Can you work these out from the model? Positions are in its coordinate system, mm. Face numbers are marked on the shaded views. A direction names the side the tool comes from. Give positions to 0.01 mm unless a question says otherwise; leave off trailing zeros. Write each loop counter-clockwise with the first axis right and the second up, starting at its lowest first coordinate (ties: lowest second). Pieces come first, ordered by that corner, then holes.
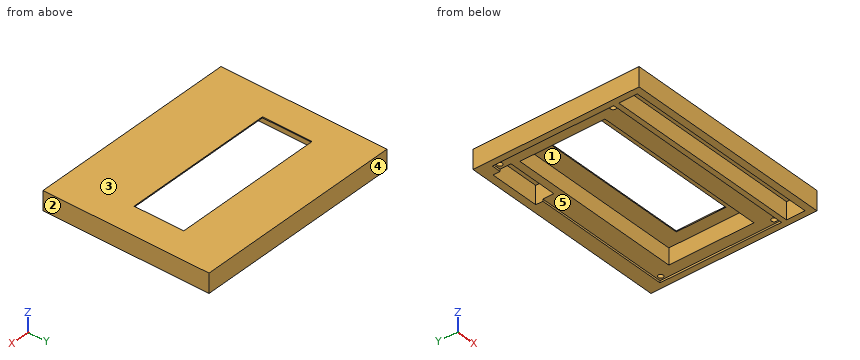
```python
from build123d import *

# Parameters (mm, degrees)
F1_W     = 104
F1_H     = 82
F1_W_2   = 87
F1_H_2   = 42
F1_W_3   = 75
F1_H_3   = 24.5
F1_W_4   = 25
F1_H_4   = 5.41
F1_H_5   = 3.5
F2_DEPTH = 9.5
F3_DEPTH = 9
F4_DEPTH = 1
F0_R     = 1.25
F5_DEPTH = 4
F6_W     = 98
F6_H     = 9.1468319297
F7_DEPTH = 8.5


with BuildPart() as f2:
    # F1 (on Top) → F2 (new body)
    with BuildSketch(Plane.XY):
        with Locations((0, -4)):
            Rectangle(F1_W, F1_H)
        Polygon((-44.4778376818, 30), (-44.4778376818, 33.5), (-19.4778376818, 33.5), (-19.4778376818, 30), (49, 30), (49, -30), (-49, -30), (-49, 30), align=None, mode=Mode.SUBTRACT)
        Polygon((-44.4778376818, 24.59), (-44.4778376818, 30), (-49, 30), (-49, -30), (49, -30), (49, 30), (-19.4778376818, 30), (-19.4778376818, 24.59), align=None)
        Rectangle(F1_W_2, F1_H_2, mode=Mode.SUBTRACT)
        Rectangle(F1_W_2, F1_H_2)
        Rectangle(F1_W_3, F1_H_3, mode=Mode.SUBTRACT)
        with Locations((-31.9778376818, 27.295)):
            Rectangle(F1_W_4, F1_H_4)
        with Locations((-31.9778376818, 31.75)):
            Rectangle(F1_W_4, F1_H_5)
    extrude(amount=F2_DEPTH)

    # F1 (on Top) → F3 (cut)
    with BuildSketch(Plane.XY):
        Rectangle(F1_W_2, F1_H_2)
        Rectangle(F1_W_3, F1_H_3, mode=Mode.SUBTRACT)
        with Locations((-31.9778376818, 27.295)):
            Rectangle(F1_W_4, F1_H_4)
        with Locations((-31.9778376818, 31.75)):
            Rectangle(F1_W_4, F1_H_5)
    extrude(amount=F3_DEPTH, mode=Mode.SUBTRACT)

    # F1 (on Top) → F4 (cut)
    with BuildSketch(Plane.XY):
        Polygon((-44.4778376818, 24.59), (-44.4778376818, 30), (-49, 30), (-49, -30), (49, -30), (49, 30), (-19.4778376818, 30), (-19.4778376818, 24.59), align=None)
        Rectangle(F1_W_2, F1_H_2, mode=Mode.SUBTRACT)
        Rectangle(F1_W_2, F1_H_2)
        Rectangle(F1_W_3, F1_H_3, mode=Mode.SUBTRACT)
        with Locations((-31.9778376818, 27.295)):
            Rectangle(F1_W_4, F1_H_4)
    extrude(amount=F4_DEPTH, mode=Mode.SUBTRACT)

    # F0 (on Top) → F5 (cut)
    with BuildSketch(Plane.XY):
        with Locations((-47, 28)):
            Circle(F0_R)
        with Locations((47, 28)):
            Circle(F0_R)
        with Locations((47, -28)):
            Circle(F0_R)
        with Locations((-47, -28)):
            Circle(F0_R)
    extrude(amount=F5_DEPTH, mode=Mode.SUBTRACT)

    # F6 (on face) → F7 (cut)
    with BuildSketch(Plane(origin=(0, 0, 0), x_dir=(1, 0, 0), z_dir=(0, 0, -1))):
        with Locations((0, 37.0334051549)):
            Rectangle(F6_W, F6_H)
    extrude(amount=-F7_DEPTH, mode=Mode.SUBTRACT)


solid = f2.part
```
1) Suppose I cut it at D-D on y = -25. Write out the boundary of the cut face in (x, z).
Values follow:
outline: (-52, 0) - (-49, 0) - (-49, 1) - (49, 1) - (49, 0) - (52, 0) - (52, 9.5) - (-52, 9.5) - close
2) Please list where these lines run through material, in increasing order: L1, parallel to X at y = 28, z = 2.9; L2, parallel to Y at x = 15.5, z = 1.25; L3, parallel to Y at x = -20.5, z = 1.5.
Values follow:
L1: x = -52 to -48.25, -45.75 to -44.48, -19.48 to 45.75, 48.25 to 52
L2: y = -45 to -41.61, -32.46 to -21, 21 to 37
L3: y = -45 to -41.61, -32.46 to -21, 21 to 24.59, 33.5 to 37
3) Suppose I cut it at A-A on y = -11. Write out the boundary of the cut face in (x, z), plus the area to 4 significant figures.
Values follow:
outline: (-52, 0) - (-49, 0) - (-49, 1) - (-43.5, 1) - (-43.5, 9) - (-37.5, 9) - (-37.5, 9.5) - (-52, 9.5) - close; (37.5, 9) - (43.5, 9) - (43.5, 1) - (49, 1) - (49, 0) - (52, 0) - (52, 9.5) - (37.5, 9.5) - close
area: 156.5 mm2
4) Suppose I cut it at C-C on x = 14.5. Write out the boundary of the cut face in (y, z).
Values follow:
outline: (-45, 0) - (-41.61, 0) - (-41.61, 8.5) - (-32.46, 8.5) - (-32.46, 0) - (-30, 0) - (-30, 1) - (-21, 1) - (-21, 9) - (-12.25, 9) - (-12.25, 9.5) - (-45, 9.5) - close; (12.25, 9) - (21, 9) - (21, 1) - (30, 1) - (30, 0) - (37, 0) - (37, 9.5) - (12.25, 9.5) - close
5) For the marked faces 1 and 2, which set-ups out of +Z, -Z, +X, -X, +Y, -Y let a thin tool reach every point of the face, with its end or its side?
Values follow:
face 1: -Z
face 2: +Z, -Z, +X, +Y, -Y
6) If we mould it in two halves opening along Y, with no side actions, what happens to the marked faces 3, 4 and 5? For each: +Y half, -Y half, draft (parallel to the pull), parting line (faces both ways), or undercut.
Values follow:
face 3: draft
face 4: +Y half
face 5: undercut
7) For pin 1 Ø2 at (x, y) = (47.5, 28.5) entering from -Z, with a flat end and sliding along its axis, tell me the tip position at first contact or that it passes through.
Values follow:
pin 1: stops at z = 1
8) Suppose I cut it at B-B on x = 47. Write out the boundary of the cut face in (y, z).
Values follow:
outline: (-45, 0) - (-41.61, 0) - (-41.61, 8.5) - (-32.46, 8.5) - (-32.46, 0) - (-30, 0) - (-30, 1) - (-29.25, 1) - (-29.25, 4) - (-26.75, 4) - (-26.75, 1) - (26.75, 1) - (26.75, 4) - (29.25, 4) - (29.25, 1) - (30, 1) - (30, 0) - (37, 0) - (37, 9.5) - (-45, 9.5) - close
